Build history of the part. All positions in model axes, mm. Face numbers are marked on the shaded views. A direction names the side the tool comes from. Coordinates: 2 decimals unless noted, no trailing zeros. Write each loop counter-clockwise with the first axis right and the second up, starting at its lowest first coordinate (ties: lowest second). Pieces come first, ordered by that corner, then holes. Notation, with made-up numbers: (85.25, -23) -> (120.25, -23) arc R27 ccw to (120.25, -5) -> close; hole circle Ø11 at (58, 79.5). An arc over 180 degrees is marked (long way). Write each question's results on one line, items separated by ' | '. Start each with the question number.
Q1. Saw through at C-C on z = 0.5. Give the cut face in (x, y), and give its area (3 significant figures).
Q2. Drill centre lines: line 1 (Z direction, x = 5.5, y = 0.5); line 2 (X direction, y = -1.75, z = 3.75); line 3 (Y direction, x = 0.75, z = 4.25). Where is each one in solid material? Low to high.
Q3. Saw through at B-B on y = 0.75. Give the cut face in (x, z), and give its area (3 significant figures).
Q4. Drop flat-ended pins along their axis: pin 1 Ø3.5 at (y, z) = (-3.5, 2.5) entering from +X; pin 2 Ø2 at (y, z) = (-3, 2) entering from -X. Give the stop position or say it passes through.
Q5. Tool access for the marked faces 4, 5 and 6: list every direction of +Z, -Z, +X, -X, +Y, -Y with a clear straight run to the whole face (end or side of a thin tool).
Q6. Two-plate mould, pull along Z, no slides. Class the marked faces 1, 2 and 3: released by +Z, released by -Z, zero draft, split by the parting line, or undercut.
Q7. Saw through at D-D on x = 3.75. Give the cut face in (y, z).
Q8. Saw through at A-A on x = 5.75. Give the cut face in (y, z), and give its area (3 significant figures).
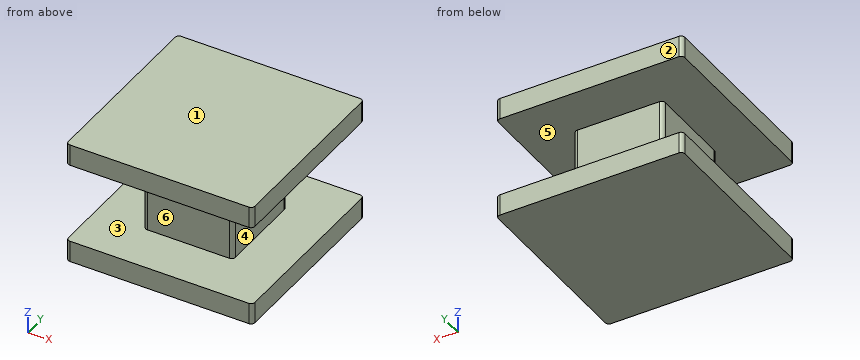
from build123d import *

# Parameters (mm, degrees)
SKETCH2_W           = 4.8
SKETCH2_H           = 4.8
BOSS_EXTRUDE1_DEPTH = 4.3
SKETCH3_W           = 10
SKETCH3_H           = 10
BOSS_EXTRUDE2_DEPTH = 1.15
SKETCH4_W           = 10
SKETCH4_H           = 10
BOSS_EXTRUDE4_DEPTH = 1.15
FILLET2_R           = 0.2


with BuildPart() as part:
    # Sketch2 → Boss-Extrude1 (new body)
    with BuildSketch(Plane.XY):
        with Locations((2.4, -2.4)):
            Rectangle(SKETCH2_W, SKETCH2_H)
    extrude(amount=BOSS_EXTRUDE1_DEPTH)

    # Sketch3 → Boss-Extrude2 (add)
    with BuildSketch(Plane.XY.offset(4.3)):
        with Locations((2.4, -2.4)):
            Rectangle(SKETCH3_W, SKETCH3_H)
    extrude(amount=BOSS_EXTRUDE2_DEPTH)

    # Sketch4 → Boss-Extrude4 (add)
    with BuildSketch(Plane(origin=(0, 0, 0), x_dir=(-1, 0, 0), z_dir=(0, 0, -1))):
        with Locations((-2.4, -2.4)):
            Rectangle(SKETCH4_W, SKETCH4_H)
    extrude(amount=BOSS_EXTRUDE4_DEPTH)

    # Fillet2
    fillet2_edges = [part.edges().sort_by_distance(p)[0] for p in [
        (-2.6, 2.6, 4.875),
        (-2.6, -7.4, 4.875),
        (7.4, -7.4, 4.875),
        (7.4, 2.6, 4.875),
        (7.4, 2.6, -0.575),
        (7.4, -7.4, -0.575),
        (-2.6, -7.4, -0.575),
        (-2.6, 2.6, -0.575),
        (0, 0, 2.15),
        (4.8, 0, 2.15),
        (4.8, -4.8, 2.15),
        (0, -4.8, 2.15),
    ]]
    fillet(fillet2_edges, radius=FILLET2_R)


solid = part.part
Returned:
1) outline: (0, -4.6) arc R0.2 ccw to (0.2, -4.8) -> (4.6, -4.8) arc R0.2 ccw to (4.8, -4.6) -> (4.8, -0.2) arc R0.2 ccw to (4.6, 0) -> (0.2, 0) arc R0.2 ccw to (0, -0.2) -> close | area: 23.0 mm2
2) line 1: z = -1.15 to 0, 4.3 to 5.45 | line 2: x = 0 to 4.8 | line 3: y = -4.8 to 0
3) outline: (-2.6, -1.15) -> (7.4, -1.15) -> (7.4, 0) -> (-2.6, 0) -> close; (-2.6, 4.3) -> (7.4, 4.3) -> (7.4, 5.45) -> (-2.6, 5.45) -> close | area: 23.0 mm2
4) pin 1: stops at x = 4.8 | pin 2: stops at x = 0
5) face 4: +X, +Y, -Y | face 5: none | face 6: +X, -X, -Y
6) face 1: released by +Z | face 2: zero draft | face 3: undercut
7) outline: (-7.4, -1.15) -> (2.6, -1.15) -> (2.6, 0) -> (0, 0) -> (0, 4.3) -> (2.6, 4.3) -> (2.6, 5.45) -> (-7.4, 5.45) -> (-7.4, 4.3) -> (-4.8, 4.3) -> (-4.8, 0) -> (-7.4, 0) -> close
8) outline: (-7.4, -1.15) -> (2.6, -1.15) -> (2.6, 0) -> (-7.4, 0) -> close; (-7.4, 4.3) -> (2.6, 4.3) -> (2.6, 5.45) -> (-7.4, 5.45) -> close | area: 23.0 mm2
